Autodesk Inventor part; units mm, degrees
ref_plane "YZ Plane" through (0, 0, 0) normal (1, 0, 0) x (0, 1, 0)
ref_plane "XZ Plane" through (0, 0, 0) normal (0, 1, 0) x (-1, 0, 0)
ref_plane "XY Plane" through (0, 0, 0) normal (0, 0, 1) x (1, 0, 0)
sketch "Sketch1" plane through (0, 0, 0) normal (0, 1, 0) x (-1, 0, 0)
  line L0 (6.35, 3.6662) -> (6.35, -3.6662)
  line L1 (6.35, -3.6662) -> (0, -7.3323)
  line L2 (0, -7.3323) -> (-6.35, -3.6662)
  line L3 (-6.35, -3.6662) -> (-6.35, 3.6662)
  line L4 (-6.35, 3.6662) -> (0, 7.3323)
  line L5 (0, 7.3323) -> (6.35, 3.6662)
  point P0 (0, 0)
  point P1 (0, 0)
  point P2 (-6.35, 0)
  point P3 (6.35, 0)
  dimension "d0" = 12.7
extrude "Extrusion1" add sketch "Sketch1" along normal blind 304.8
sketch "Sketch2" plane through (0, 304.8, 0) normal (0, 1, 0) x (1, 0, 0)
  circle A0 centre (0, 0) radius 2.5527
  dimension "d3" = 5.1054
extrude "Extrusion2" cut sketch "Sketch2" against normal blind 50.8
sketch "Sketch3" plane through (0, 0, 0) normal (0, -1, 0) x (1, 0, 0)
  circle A0 centre (0, 0) radius 2.5527
  dimension "d6" = 5.1054
extrude "Extrusion3" cut sketch "Sketch3" against normal blind 50.8
thread "Thread1"
properties part number "CORL_003_Shaft" material "Aluminum 6061"
Read the model definition and answer for the solid it produces. Units are mm, in the model's axes. A direction names the side the tool comes from. Round coordinates to 2 decimals unless told otherwise and drop trailing zeros. Write each loop counter-clockwise with the first axis right and the second up, starting at its lowest first coordinate (ties: lowest second). Pieces come first, ordered by that corner, then holes. Notation, with made-up numbers: M -18.75,77.5 L -0.75,77.5 A10 cw -0.75,93.5 Z; hole C -18.5,64.5 d10. An arc over 180 degrees is marked long. One line per item, written item: value.
Q1. Flat-ended cylindrical pins translate along their axes: pin 1 Ø2.5 at (x, z) = (-1, 0.5) entering from -Y; pin 2 Ø2 at (x, y) = (2.5, 55.5) entering from +Z; pin 3 Ø1.5 at (y, z) = (87, -5.5) entering from +X. Find the tip coordinate at first contact, or state that the pin passes through.
Data:
pin 1: y = 50.8
pin 2: z = 6.47
pin 3: x = 4.47
Q2. Find section C-C on y = 131. Write down the section's boundary in (x, z).
Data:
outline: M -6.35,-3.67 L 0,-7.33 L 6.35,-3.67 L 6.35,3.67 L 0,7.33 L -6.35,3.67 Z
Q3. Find section B-B on z = 0. Write down the section's boundary in (x, y).
Data:
outline: M -6.35,0 L -2.55,0 L -2.55,50.8 L 2.55,50.8 L 2.55,0 L 6.35,0 L 6.35,304.8 L 2.55,304.8 L 2.55,254 L -2.55,254 L -2.55,304.8 L -6.35,304.8 Z
Q4. Straight lines are drawn through the part: line 1 (Z direction, x = 0, y = 283); line 2 (Z direction, x = 2.25, y = 41); line 3 (X direction, y = 293.5, z = 0). For each, find the intervals that lie inside material, in ascending order. Write a range as [from, to].
Data:
line 1: [-7.33, -2.55], [2.55, 7.33]
line 2: [-6.03, -1.21], [1.21, 6.03]
line 3: [-6.35, -2.55], [2.55, 6.35]
Q5. Which of the six approach directions +Z, -Z, +X, -X, +Y, -Y give full straight-line access (tool end or side, diameter ignored) to faces 1 (the flat face through (-3.219, 150.266, -5.474)), 2 (the cylindrical face through (2.435, 25.044, 0.767))?
Data:
face 1: -Z, -X, +Y, -Y
face 2: -Y
Q6. Find section A-A on y = 283. Write down the section's boundary in (x, z).
Data:
outline: M -6.35,-3.67 L 0,-7.33 L 6.35,-3.67 L 6.35,3.67 L 0,7.33 L -6.35,3.67 Z; hole C 0,0 d5.11
Q7. For a pull along X with two mould halves and no side action, classify faces 3 (the flat face through (-3.131, 150.266, 5.525)), 4 (the cylindrical face through (2.435, 279.756, -0.767)), 5 (the flat face through (0, 254, 0)), 6 (the flat face through (0, 304.8, -3)) as +X half, -X half, draft (parallel to the pull), parting line (faces both ways), or undercut.
Data:
face 3: -X half
face 4: undercut
face 5: undercut
face 6: draft
